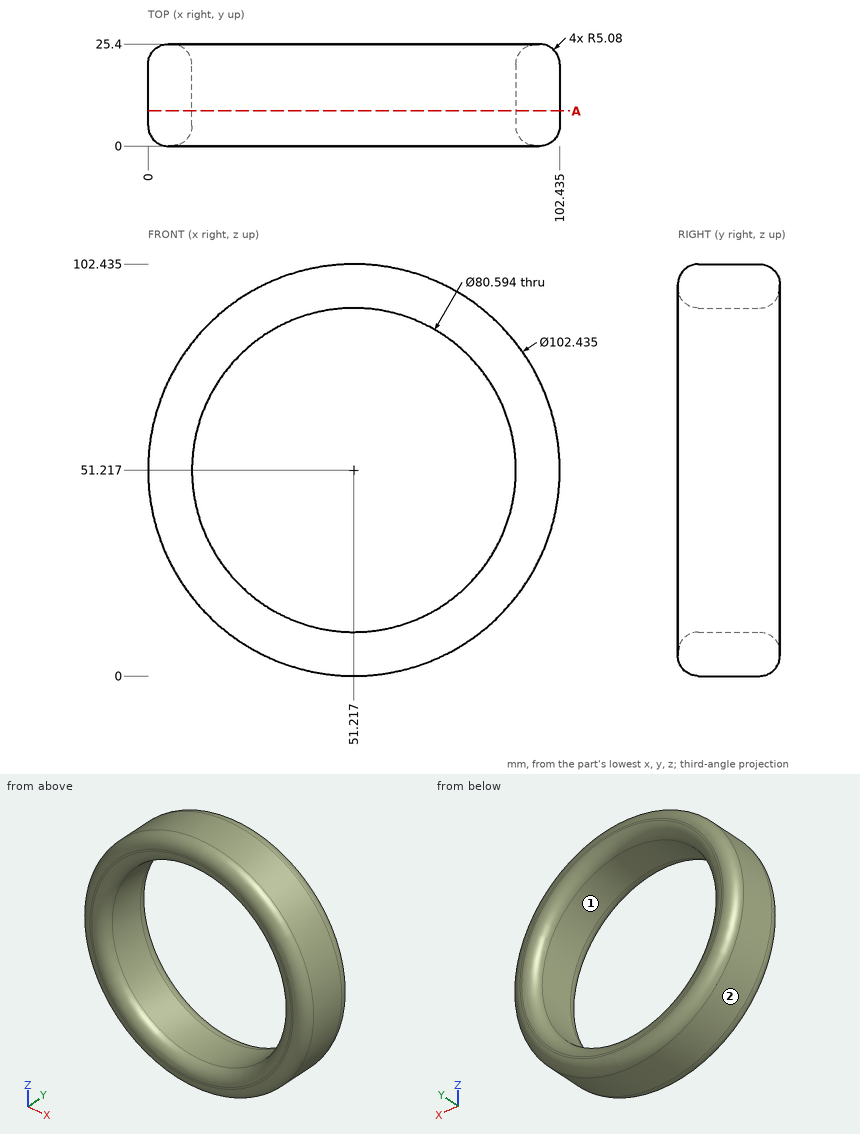
Could you check a few things on this drawing? It's one solid part, dimensions in mm from its lowest x, y, z. Give positions to 0.01 mm unless a question says otherwise; leave off trailing zeros. Write each loop counter-clockwise with the first axis right and the second up, starting at its lowest first coordinate (ties: lowest second). Pieces come first, ordered by that corner, then holes.
(1) Will these pins go through, and if not, where does the flat tip stop? pin 1 (1 mm diameter, centred on y = 21, z = 36.5, fed in from -X); pin 2 (2 mm diameter, centred on x = 44.5, y = 20, fed in from -Z); pin 3 (1 mm diameter, centred on y = 14.5, z = 19, fed in from -X); pin 4 (10 mm diameter, centred on y = 17.5, z = 51, fed in from -X).
Output values:
pin 1: stops at x = 2.05
pin 2: stops at z = 0.32
pin 3: stops at x = 11
pin 4: stops at x = 0
(2) If I drill on L1, parallel to X at y = 2, z = 75.5 (1 decimal); L2, parallel to Z at x = 24, y = 19.5 (1 decimal); L3, parallel to Z at x = 79.5, y = 17.5 (1 decimal), over which ranges is the centre line in solid material (lowest first)?
Output values:
L1: x = 7.3 to 17.8, 84.7 to 95.1
L2: z = 7.8 to 21.5, 80.9 to 94.6
L3: z = 8.5 to 22.5, 79.9 to 93.9
(3) Imagine slicing it at A-A, the plane y = 8.75. Write out the boundary of the cut face in (x, z) (1 decimal).
Output values:
outline: circle Ø102.4 at (51.2, 51.2); hole circle Ø80.6 at (51.2, 51.2)
(4) Thinking about a two-plate mould opening in Z: for the marked faces 1 and 2, which applies, pulls with the +Z half, pulls with the -Z half, needs draft (parallel to the pull), parting line crosses it, or undercut?
Output values:
face 1: undercut
face 2: parting line crosses it
